Here's how the part is built. I have some questions about the finished solid (model axes, mm). A direction names the side the tool comes from. Coordinates: 2 decimals unless noted, no trailing zeros. Write each loop counter-clockwise with the first axis right and the second up, starting at its lowest first coordinate (ties: lowest second). Pieces come first, ordered by that corner, then holes.
Item 1: I want a section at A-A (z = 62). Please give me the cut outline in (x, y).
Item 2: I want a section at B-B (y = -10.5). Please give me the cut outline in (x, z).
Item 3: I want a section at D-D (z = 48.5). Please give me the cut outline in (x, y).
Item 4: If we mould it in two halves opening along X, with no side actions, what happens to faces 1 (the face through (39.7, 10.21, 74.87)), 2 (the face through (-51, -4, 10)), 3 (the face through (-11, 7, 90))? For each: pulls with the +X half, pulls with the -X half, needs draft (parallel to the pull), parting line crosses it, or undercut.
Item 5: For faces 4 (the face through (-1.77, 0.12, 10)), 5 (the face through (-6, 4, 0)), which set-ups out of +Z, -Z, +X, -X, +Y, -Y let a thin tool reach every point of the face, with its end or its side?
Item 6: Please list where these lines run through material, in increasing order: line 1 (X direction, y = 0, z = 23.5); line 2 (Z direction, x = 36, y = 4); line 3 (Y direction, x = -50.5, z = 51).
Item 7: I'm going to push flat-ended pins straight in: P1, Ø15.5, axis at x = 39.57, y = 0, coming from the +Z side; P2, Ø8.5, axis at x = 36.5, y = -3.5, coming from the +Z side; P3, Ø8, axis at x = 24, y = 5, coming from the +Z side. Where does each tip first touch, or does it pass through?
Item 8: I want a section at C-C (x = 41.5). Please give me the cut outline in (y, z).
from build123d import *

# Parameters (mm, degrees)
F0_W            = 120
F0_H            = 30
F0_R            = 3.5
F1_DEPTH        = 10
F2_W            = 120
F2_H            = 30
F2_R            = 8.5
F3_DEPTH        = 80
F4_R            = 25.5
F5_DEPTH        = 30
F6_T1_DEPTH     = 184.300979278
F7_SIZE         = 8
F10_D           = 5
F10_DEPTH       = 25
F10_TIP         = 1.5021515476
F10_ON_F9_D     = 5
F10_ON_F9_DEPTH = 25
F10_ON_F9_TIP   = 1.5021515476


# Not quite as in the source:
# - a fillet or chamfer that OpenCascade refuses, or shapes differently, is made with other operations: its cross-section is extruded or revolved along the edge and cut away or added


with BuildPart() as f1:
    # F0 (on Top) → F1 (new body)
    with BuildSketch(Plane.XY):
        with Locations((-5.4327639937, 0)):
            Rectangle(F0_W, F0_H)
        with Locations((-50.4327639937, 0)):
            Circle(F0_R, mode=Mode.SUBTRACT)
        with Locations((-5.4327639937, 0)):
            Circle(F0_R, mode=Mode.SUBTRACT)
        with Locations((39.5672360063, 0)):
            Circle(F0_R, mode=Mode.SUBTRACT)
    extrude(amount=F1_DEPTH)

    # F2 (on face) → F3 (join)
    with BuildSketch(Plane.XY.offset(10)):
        with Locations((-5.4327639937, 0)):
            Rectangle(F2_W, F2_H)
        with Locations((-50.4327639937, 0)):
            Circle(F2_R, mode=Mode.SUBTRACT)
        with Locations((-5.4327639937, 0)):
            Circle(F2_R, mode=Mode.SUBTRACT)
        with Locations((39.5672360063, 0)):
            Circle(F2_R, mode=Mode.SUBTRACT)
    extrude(amount=F3_DEPTH)

    # F4 (on face) → F5 (cut)
    with BuildSketch(Plane.XZ.offset(15)):
        with Locations((-5.4327639937, 55)):
            Circle(F4_R)
    extrude(amount=-F5_DEPTH, mode=Mode.SUBTRACT)

    # F6: chamfer of 30 on 2 edges, made by hand

    # F6_s2 → F6_t1 (cut)
    with BuildSketch(Plane.XZ.offset(-92.150489639)):
        Polygon((-35.4327639937, 90), (-65.4327639937, 60), (-65.4327639937, 90), align=None)
        Polygon((54.5672360063, 60), (24.5672360063, 90), (54.5672360063, 90), align=None)
    extrude(amount=F6_T1_DEPTH, mode=Mode.SUBTRACT)

    # F7
    f7_edges = [f1.edges().sort_by_distance(p)[0] for p in [
        (-65.432764, 0, 60),
        (-35.432764, 0, 90),
        (24.567236, 0, 90),
        (54.567236, 0, 60),
    ]]
    chamfer(f7_edges, length=F7_SIZE)

    # F10
    with Locations(Plane(origin=(-35.8372404269, 0, 86.5187518767), x_dir=(0.9238795325, 0, 0.3826834324), z_dir=(-0.3826834324, 0, 0.9238795325))):
        with Locations((1.7059034787, 0)):
            Hole(F10_D / 2, depth=F10_DEPTH)
            with Locations((0, 0, -(F10_DEPTH + F10_TIP / 2))):  # 118° drill point
                Cone(0, F10_D / 2, F10_TIP, mode=Mode.SUBTRACT)

    # F10 on F9
    with Locations(Plane(origin=(34.2460206938, 0, 82.6772076162), x_dir=(0.9238795325, 0, -0.3826834324), z_dir=(0.3826834324, 0, 0.9238795325))):
        with Locations((-11.7443423963, 0)):
            Hole(F10_ON_F9_D / 2, depth=F10_ON_F9_DEPTH)
            with Locations((0, 0, -(F10_ON_F9_DEPTH + F10_ON_F9_TIP / 2))):  # 118° drill point
                Cone(0, F10_ON_F9_D / 2, F10_ON_F9_TIP, mode=Mode.SUBTRACT)


solid = f1.part
Answer:
1. outline: (-61.29, -15) - (-29.95, -15) - (-29.95, 15) - (-61.29, 15) - close; (19.09, -15) - (50.43, -15) - (50.43, 15) - (19.09, 15) - close; hole circle Ø17 at (-50.43, 0); hole circle Ø17 at (39.57, 0)
2. outline: (-65.43, 0) - (54.57, 0) - (54.57, 52) - (48.91, 65.66) - (30.22, 84.34) - (16.57, 90) - (-27.43, 90) - (-41.09, 84.34) - (-59.78, 65.66) - (-65.43, 52) - close; hole circle Ø51 at (-5.43, 55)
3. outline: (-65.43, -15) - (-30.09, -15) - (-30.09, 15) - (-65.43, 15) - close; (19.22, -15) - (54.57, -15) - (54.57, 15) - (19.22, 15) - close; hole circle Ø17 at (-50.43, 0); hole circle Ø17 at (39.57, 0)
4. face 1: pulls with the +X half
4. face 2: undercut
4. face 3: needs draft
5. face 4: +Z
5. face 5: -Z, +X, -X, +Y, -Y
6. line 1: x = -65.43 to -58.93, -41.93 to -13.93, 3.07 to 31.07, 48.07 to 54.57
6. line 2: z = 0 to 10
6. line 3: y = -15 to -8.5, 8.5 to 15
7. P1: stops at z = 10
7. P2: stops at z = 82.19
7. P3: stops at z = 88.58
8. outline: (-15, 0) - (-2.92, 0) - (-2.92, 10) - (-8.28, 10) - (-8.28, 73.07) - (-15, 73.07) - close; (2.92, 0) - (15, 0) - (15, 73.07) - (8.28, 73.07) - (8.28, 10) - (2.92, 10) - close
